from build123d import *

# Parameters (mm, degrees)
SKETCH1_W           = 62.7
SKETCH1_H           = 58.1
SKETCH1_R           = 25
BOSS_EXTRUDE1_DEPTH = 5
SKETCH2_R           = 1.5
BOSS_EXTRUDE2_DEPTH = 3


with BuildPart() as part:
    # Sketch1 → Boss-Extrude1 (new body)
    with BuildSketch(Plane(origin=(0, 0, 0), x_dir=(1, 0, 0), z_dir=(0, 1, 0))):
        Rectangle(SKETCH1_W, SKETCH1_H)
        with Locations(Location((0, 0, 0), (0, 0, 270))):
            Circle(SKETCH1_R, mode=Mode.SUBTRACT)
    extrude(amount=BOSS_EXTRUDE1_DEPTH)

    # Sketch2 → Boss-Extrude2 (add)
    with BuildSketch(Plane.XZ):
        with Locations(Location((-27.163407974, 24.863407974, 0), (0, 0, 270))):
            Circle(SKETCH2_R)
        with Locations(Location((27.163407974, 24.863407974, 0), (0, 0, 90))):
            Circle(SKETCH2_R)
        with Locations(Location((27.163407974, -24.863407974, 0), (0, 0, 270))):
            Circle(SKETCH2_R)
        with Locations(Location((-27.163407974, -24.863407974, 0), (0, 0, 90))):
            Circle(SKETCH2_R)
    extrude(amount=BOSS_EXTRUDE2_DEPTH)


solid = part.part
The listing builds one solid part. Answer for the finished solid, in the listing's coordinates (mm). A direction names the side the tool comes from. Round coordinates to 2 decimals unless told otherwise and drop trailing zeros. Write each loop counter-clockwise with the first axis right and the second up, starting at its lowest first coordinate (ties: lowest second). Pieces come first, ordered by that corner, then holes. Notation, with made-up numbers: M -7,49 L 10,49 A22 cw 10,85 Z; hole C 39.25,-23 d8. An arc over 180 degrees is marked long. Write each question's results on one line, items separated by ' | '. Start each with the question number.
Item 1: Straight lines are drawn through the part: probe 1 along X at (y, z) = (1.7, 0); probe 2 along Y at (x, z) = (-20, 25); probe 3 along X at (y, z) = (4.75, 7). For each, find the intervals that lie inside material, in ascending order.
Item 2: Find section A-A on z = 0. Write down the section's boundary in (x, y).
Item 3: Find section B-B on x = 0. Write down the section's boundary in (y, z).
Item 4: Which of the six approach directions +Z, -Z, +X, -X, +Y, -Y give full straight-line access (tool end or side, diameter ignored) to faces 1 (the cylindrical face through (28.63, -1.48, 24.54)), 2 (the flat face through (27, -3, 25))?
Item 5: Find section C-C on y = 1.25. Write down the section's boundary in (x, z).
Item 6: The mould has two halves that part along Z. Classify faces 3 (the flat face through (-31.35, 2, 0)), 4 (the cylindrical face through (-28.628, -1.479, 25.189)), 5 (the flat face through (0, 2, 29.05)), 6 (the cylindrical face through (7.509, 2.465, 23.846)): +Z half, -Z half, draft (parallel to the pull), parting line (faces both ways), or undercut.
Answer block:
1) probe 1: x = -31.35 to -25, 25 to 31.35 | probe 2: y = 0 to 5 | probe 3: x = -31.35 to -24, 24 to 31.35
2) outline: M -31.35,0 L -25,0 L -25,5 L -31.35,5 Z; M 25,0 L 31.35,0 L 31.35,5 L 25,5 Z
3) outline: M 0,-29.05 L 5,-29.05 L 5,-25 L 0,-25 Z; M 0,25 L 5,25 L 5,29.05 L 0,29.05 Z
4) face 1: -Y | face 2: +Z, -Z, +X, -X, -Y
5) outline: M -31.35,-29.05 L 31.35,-29.05 L 31.35,29.05 L -31.35,29.05 Z; hole C 0,0 d50
6) face 3: draft | face 4: undercut | face 5: +Z half | face 6: undercut
